Autodesk Inventor part; units mm, degrees
ref_plane "YZ Plane" through (0, 0, 0) normal (1, 0, 0) x (0, 1, 0)
ref_plane "XZ Plane" through (0, 0, 0) normal (0, 1, 0) x (-1, 0, 0)
ref_plane "XY Plane" through (0, 0, 0) normal (0, 0, 1) x (1, 0, 0)
sketch "스케치1" plane through (0, 0, 0) normal (0, 0, 1) x (1, 0, 0)
  line L0 (7.5, 38) -> (7.5, 36.5)
  line L1 (2, 38) -> (7.5, 38)
  line L2 (2, 38) -> (2, 8)
  line L3 (2, 8) -> (6.525, 8)
  line L4 (6.525, 10.5) -> (6.525, 8)
  line L5 (6.525, 10.5) -> (10.3997, 10.5)
  line L6 (10.3997, 10.5) -> (10.6003, 10.5)
  line L7 (10.6003, 10.5) -> (14.475, 10.5)
  line L8 (14.475, 10.5) -> (14.475, 8)
  line L9 (14.475, 8) -> (28.525, 8)
  line L10 (28.525, 10.5) -> (28.525, 8)
  line L11 (28.525, 10.5) -> (32.3997, 10.5)
  line L12 (32.3997, 10.5) -> (32.6003, 10.5)
  line L13 (32.6003, 10.5) -> (34.7876, 10.5)
  line L14 (34.7876, 10.5) -> (34.7876, 19.4)
  line L15 (36, 19.4) -> (34.7876, 19.4)
  line L16 (36, 24) -> (36, 19.4)
  line L17 (38.55, 24) -> (36, 24)
  line L18 (38.55, 24) -> (38.55, 25.4)
  line L19 (38.55, 25.4) -> (37.1, 25.4)
  line L20 (37.1, 25.4) -> (37.1, 35.5)
  line L21 (49.9, 35.5) -> (37.1, 35.5)
  line L22 (49.9, 25.4) -> (49.9, 35.5)
  line L23 (49.9, 25.4) -> (48.45, 25.4)
  line L24 (48.45, 24) -> (48.45, 25.4)
  line L25 (51, 24) -> (48.45, 24)
  line L26 (51, 24) -> (51, 10.5)
  line L27 (51, 10.5) -> (54.3997, 10.5)
  line L28 (54.3997, 10.5) -> (54.6003, 10.5)
  line L29 (54.6003, 10.5) -> (57.5, 10.5)
  line L30 (57.5, 36.5) -> (57.5, 10.5)
  line L31 (57.5, 36.5) -> (51.5, 36.5)
  line L32 (51.5, 38) -> (51.5, 36.5)
  line L33 (35.5, 38) -> (51.5, 38)
  line L34 (35.5, 36.5) -> (35.5, 38)
  line L35 (35.5, 36.5) -> (29.5, 36.5)
  line L36 (29.5, 38) -> (29.5, 36.5)
  line L37 (13.5, 38) -> (29.5, 38)
  line L38 (13.5, 36.5) -> (13.5, 38)
  line L39 (13.5, 36.5) -> (7.5, 36.5)
  line L40 (22.05, 14.2) -> (27.95, 14.2)
  line L41 (22.05, 18) -> (22.05, 14.2)
  line L42 (27.95, 18) -> (22.05, 18)
  line L43 (27.95, 14.2) -> (27.95, 18)
  line L44 (34.6876, 10.6) -> (7.6, 10.6)
  line L45 (7.6, 10.6) -> (7.6, 36.4)
  line L46 (7.6, 36.4) -> (34.6876, 36.4)
  line L47 (34.6876, 36.4) -> (34.6876, 10.6)
  line L48 (7.6, 36.4) -> (6.525, 36.4)
  line L49 (7.6, 10.6) -> (6.525, 10.6)
  line L50 (6.525, 10.6) -> (6.525, 36.4)
  line L51 (6.525, 36.4) -> (7.6, 36.4)
  line L52 (7.6, 36.4) -> (7.6, 10.6)
  point P0 (0, 0)
extrude "돌출1" add sketch "스케치1" along normal blind 15 contours L41 L42 L43 L40 | L44 L45 L46 L47 | L49 L50 L48 L45
sketch "스케치2" plane through (0, 0, 15) normal (0, 0, 1) x (1, 0, 0)
  line L0 (34.5, 38) -> (52.5, 38)
  line L1 (52.5, 38) -> (52.5, 36.5)
  line L2 (56.5, 36.5) -> (52.5, 36.5)
  line L3 (56.5, 38) -> (56.5, 36.5)
  line L4 (56.5, 38) -> (59.1, 38)
  line L5 (59.1, 38) -> (59.1, 40)
  line L6 (6, 40) -> (59.1, 40)
  line L7 (6, 38) -> (6, 40)
  line L8 (6, 38) -> (8.5, 38)
  line L9 (8.5, 38) -> (8.5, 36.5)
  line L10 (12.5, 36.5) -> (8.5, 36.5)
  line L11 (12.5, 38) -> (12.5, 36.5)
  line L12 (12.5, 38) -> (30.5, 38)
  line L13 (30.5, 38) -> (30.5, 36.5)
  line L14 (34.5, 36.5) -> (30.5, 36.5)
  line L15 (34.5, 38) -> (34.5, 36.5)
  line L16 (14.475, 10.5) -> (12.975, 10.5)
  line L17 (12.975, 10.5) -> (12.975, 8.5)
  line L18 (12.975, 8.5) -> (8.025, 8.5)
  line L19 (8.025, 10.5) -> (8.025, 8.5)
  line L20 (8.025, 10.5) -> (6.525, 10.5)
  line L21 (6.525, 10.5) -> (6.525, 8)
  line L22 (6, 8) -> (6.525, 8)
  line L23 (6, 8) -> (6, 6)
  line L24 (6, 6) -> (59.1, 6)
  line L25 (59.1, 8) -> (59.1, 6)
  line L26 (58.475, 8) -> (59.1, 8)
  line L27 (58.475, 8) -> (58.475, 10.5)
  line L28 (58.475, 10.5) -> (56.975, 10.5)
  line L29 (56.975, 10.5) -> (56.975, 8.5)
  line L30 (56.975, 8.5) -> (52.025, 8.5)
  line L31 (52.025, 10.5) -> (52.025, 8.5)
  line L32 (52.025, 10.5) -> (50.525, 10.5)
  line L33 (50.525, 10.5) -> (50.525, 8)
  line L34 (36.475, 8) -> (50.525, 8)
  line L35 (36.475, 8) -> (36.475, 10.5)
  line L36 (36.475, 10.5) -> (34.975, 10.5)
  line L37 (34.975, 10.5) -> (34.975, 8.5)
  line L38 (34.975, 8.5) -> (30.025, 8.5)
  line L39 (30.025, 10.5) -> (30.025, 8.5)
  line L40 (30.025, 10.5) -> (28.525, 10.5)
  line L41 (28.525, 10.5) -> (28.525, 8)
  line L42 (14.475, 8) -> (28.525, 8)
  line L43 (14.475, 8) -> (14.475, 10.5)
  line L44 (14.475, 36.4) -> (28.525, 36.4)
  line L45 (34.6876, 10.6) -> (34.6876, 36.4)
  line L46 (14.475, 10.6) -> (28.525, 10.6)
  line L47 (28.525, 10.6) -> (28.525, 36.4)
  line L48 (28.525, 36.4) -> (14.475, 36.4)
  line L49 (-13.0231, 23) -> (78.1205, 23)
  line L50 (14.5, -11.1) -> (14.5, 56.1)
  line L51 (34.6876, 36.4) -> (6.525, 36.4)
  line L52 (6.525, 36.4) -> (6.525, 10.6)
  line L53 (6.525, 10.6) -> (34.6876, 10.6)
  line L54 (28.525, 23) -> (34.6876, 23)
  line L55 (34.6876, 23) -> (34.6876, 31)
  line L56 (34.6876, 31) -> (28.525, 31)
  line L57 (28.525, 31) -> (28.525, 23)
  line L58 (28.525, 23) -> (34.6876, 23)
  line L59 (34.6876, 23) -> (34.6876, 15)
  line L60 (34.6876, 15) -> (28.525, 15)
  line L61 (28.525, 15) -> (28.525, 23)
  line L62 (6.525, 23) -> (12.688, 23)
  line L63 (12.688, 23) -> (12.688, 31)
  line L64 (12.688, 31) -> (6.525, 31)
  line L65 (6.525, 31) -> (6.525, 23)
  line L66 (14.5, 57.1) -> (14.5, -10.1)
  line L67 (12.688, 23) -> (12.688, 15)
  line L68 (12.688, 15) -> (6.525, 15)
  line L69 (6.525, 15) -> (6.525, 23)
  line L70 (6.525, 36.4) -> (6.525, 10.6)
  line L71 (12.688, 23) -> (6.525, 23)
  line L72 (6.525, 23) -> (6.525, 26)
  line L73 (6.525, 26) -> (12.688, 26)
  line L74 (12.688, 26) -> (12.688, 23)
  line L75 (12.688, 23) -> (6.525, 23)
  line L76 (6.525, 23) -> (6.525, 20)
  line L77 (6.525, 20) -> (12.688, 20)
  line L78 (12.688, 20) -> (12.688, 23)
  point P0 (0, 0)
  dimension "d3" = 6.163
  dimension "d4" = 8
extrude "돌출2" cut sketch "스케치2" against normal up to next contours L56 L45 L49 L47 | L49 L45 L60 L47 | L64 L63 L73 L52 | L67 L68 L52 L77
sketch "스케치4" plane through (6.525, 10.6, 0) normal (0, -1, 0) x (1, 0, 0)
  circle A0 centre (3.975, 2.8) radius 1.35
  circle A1 centre (25.975, 2.8) radius 1.35
  circle A2 centre (25.975, 2.8) radius 1.55
  circle A3 centre (3.975, 2.8) radius 1.55
  point P0 (-6.525, 0)
  dimension "d14" = 0.2
  dimension "d15" = 0.2
extrude "돌출4" cut sketch "스케치4" against normal up to next contours A0 | A1
sketch "스케치5" plane through (6.525, 36.4, 0) normal (0, 1, 0) x (1, 0, 0)
  circle A0 centre (25.975, -2.8) radius 1.025
  circle A1 centre (3.975, -2.8) radius 1.025
  circle A2 centre (25.975, -2.8) radius 1.225
  circle A3 centre (3.975, -2.8) radius 1.225
  point P0 (-6.525, 0)
  dimension "d16" = 0.2
  dimension "d17" = 0.2
extrude "돌출5" cut sketch "스케치5" against normal up to next contours A0 | A1
sketch "스케치6" plane through (0, 0, 0) normal (0, 0, -1) x (-1, 0, 0)
  line L0 (-28.525, 31) -> (-34.6876, 31)
  line L1 (-34.6876, 31) -> (-34.6876, 36.4)
  line L2 (-34.6876, 36.4) -> (-6.525, 36.4)
  line L3 (-6.525, 36.4) -> (-6.525, 31)
  line L4 (-6.525, 31) -> (-12.688, 31)
  line L5 (-12.688, 31) -> (-12.688, 26)
  line L6 (-12.688, 26) -> (-6.525, 26)
  line L7 (-6.525, 26) -> (-6.525, 20)
  line L8 (-6.525, 20) -> (-12.688, 20)
  line L9 (-12.688, 20) -> (-12.688, 15)
  line L10 (-12.688, 15) -> (-6.525, 15)
  line L11 (-6.525, 15) -> (-6.525, 10.6)
  line L12 (-6.525, 10.6) -> (-34.6876, 10.6)
  line L13 (-34.6876, 10.6) -> (-34.6876, 15)
  line L14 (-34.6876, 15) -> (-28.525, 15)
  line L15 (-28.525, 15) -> (-28.525, 31)
  line L16 (-12.688, 31) -> (-28.525, 31)
  line L17 (-28.525, 31) -> (-28.525, 15)
  line L18 (-28.525, 15) -> (-12.688, 15)
  line L19 (-12.688, 15) -> (-12.688, 31)
  line L20 (13.0231, 24) -> (-78.1205, 24)
  line L21 (-14.5, 58.1) -> (-14.5, -9.1)
  point P0 (0, 0)
extrude "돌출6" cut sketch "스케치6" against normal blind 7.5 contours L16 L21 L20 L15 | L20 L21 L18 L15 | L16 L5 L19 L20 L21 | L20 L19 L9 L18 L21 | L20 L7 L8 L19 | L19 L6 L7 L20
sketch "스케치7" plane through (0, 0, 15) normal (0, 0, 1) x (1, 0, 0)
  circle A0 centre (14.5, 24) radius 1.55
  point P0 (0, 0)
extrude "돌출7" cut sketch "스케치7" against normal up to next
properties part number "foot_bridge"
Read the model definition and answer for the solid it produces. Units are mm, in the model's axes. A direction names the side the tool comes from. Round coordinates to 2 decimals unless told otherwise and drop trailing zeros. Write each loop counter-clockwise with the first axis right and the second up, starting at its lowest first coordinate (ties: lowest second). Pieces come first, ordered by that corner, then holes.
Q1. Find section B-B on y = 24. Determine the outline of the cut face in (x, z) (3 decimals).
Values:
outline: (6.525, 7.5) - (12.95, 7.5) - (12.95, 15) - (6.525, 15) - close; (16.05, 7.5) - (28.525, 7.5) - (28.525, 15) - (16.05, 15) - close
Q2. Find section D-D on z = 8. Determine the outline of the cut face in (x, y) (3 decimals).
Values:
outline: (6.525, 10.6) - (34.688, 10.6) - (34.688, 15) - (28.525, 15) - (28.525, 31) - (34.688, 31) - (34.688, 36.4) - (6.525, 36.4) - (6.525, 31) - (12.688, 31) - (12.688, 26) - (6.525, 26) - (6.525, 20) - (12.688, 20) - (12.688, 15) - (6.525, 15) - close; hole circle Ø3.1 at (14.5, 24)
Q3. A tool of negligible diameter and unlimited length cuts with its end or side. For faces 1 (the face through (21, 15, 6)), 2 (the face through (20, 23, 7.5)), 3 (the face through (11.226, 12.769, 3.938)), from which of +Z, -Z, +X, -X, +Y, -Y can it reach the whole face along a straight path? Write none if from no direction.
Values:
face 1: -Z
face 2: -Z, +X, -X
face 3: -Y
Q4. The mould has two halves that part along Y. Classify faces 4 (the face through (28.525, 23, 11)), 5 (the face through (12.688, 18, 11)), 6 (the face through (21, 10.6, 7)), 7 (the face through (20, 24, 15)): released by +Y, released by -Y, zero draft, split by the parting line, or undercut.
Values:
face 4: undercut
face 5: undercut
face 6: released by -Y
face 7: zero draft
Q5. Flat-ended cylindrical pins translate along their axes: P1, Ø2.5, axis at x = 32.5, z = 2.8, coming from the -Y side; P2, Ø2.5, axis at y = 18.5, z = 12, coming from the -X side; P3, Ø6, axis at y = 22.5, z = 10, coming from the +X side (3 decimals). Find the tip coordinate at first contact, or state that the pin passes through.
Values:
P1: stops at y = 31
P2: stops at x = 12.69
P3: stops at x = 28.525
Q6. Straight lines are drawn through the part: line 1 (Y direction, x = 11, z = 10.5); line 2 (Z direction, x = 32.5, y = 35.1) (3 decimals); line 3 (Z direction, x = 10.5, y = 13.05). For each, find the intervals that lie inside material, in ascending order.
Values:
line 1: y = 10.6 to 15, 20 to 26, 31 to 36.4
line 2: z = 0 to 1.775, 3.825 to 15
line 3: z = 0 to 1.45, 4.15 to 15
Q7. Find section C-C on x = 30.75. Determine the outline of the cut face in (y, z).
Values:
outline: (10.6, 0) - (15, 0) - (15, 15) - (10.6, 15) - close; (31, 0) - (36.4, 0) - (36.4, 15) - (31, 15) - close
Q8. Find section A-A on z = 2.8. Determine the outline of the cut face in (x, y) (3 decimals).
Values:
outline: (6.525, 10.6) - (9.15, 10.6) - (9.15, 15) - (6.525, 15) - close; (6.525, 31) - (9.475, 31) - (9.475, 36.4) - (6.525, 36.4) - close; (11.525, 31) - (31.475, 31) - (31.475, 36.4) - (11.525, 36.4) - close; (11.85, 10.6) - (31.15, 10.6) - (31.15, 15) - (11.85, 15) - close; (33.525, 31) - (34.688, 31) - (34.688, 36.4) - (33.525, 36.4) - close; (33.85, 10.6) - (34.688, 10.6) - (34.688, 15) - (33.85, 15) - close
